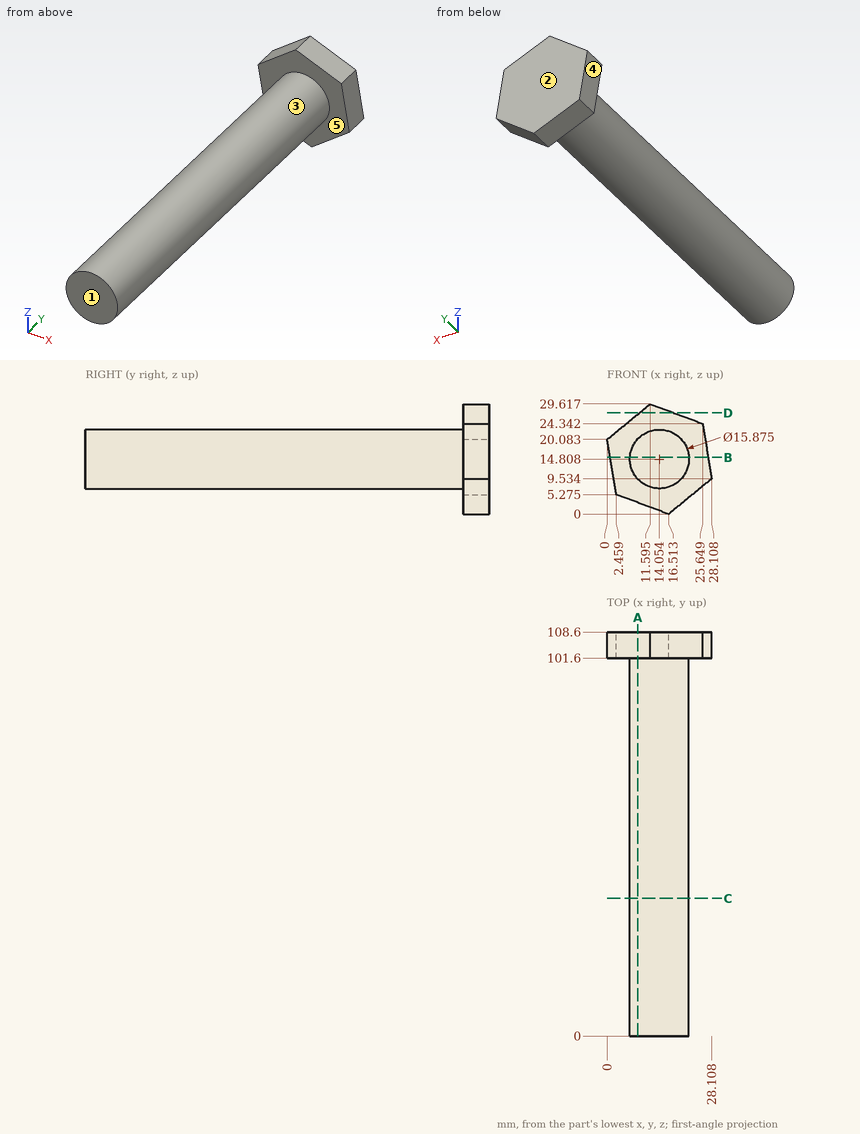
Drawing for the job (mm, zero at the part's lowest x, y, z). A direction names the side the tool comes from. Give positions to 0.01 mm unless a question says otherwise; leave off trailing zeros. Order: outer loops, then holes, each group sorted by start corner. A loop starts at its lowest first (then second) coordinate and runs counter-clockwise, first axis right, second up. Notation, with made-up numbers: M 71.5,4.25 L 76.5,4.25 A26 ccw 76.5,27.25 Z; hole C 66.5,74 d9. An arc over 180 degrees is marked long. Put each result on its own line as item: value.
Item 1: Probe line 1 (Y direction, x = 14.25, z = 28); line 2 (Z direction, x = 14, y = 13) (1 decimal); line 3 (Z direction, x = 18.5, y = 28) (1 decimal). List the from-to ranges inside material, lowest first. Write a range as [from, to].
From the geometry:
line 1: y = [101.6, 108.6]
line 2: z = [6.9, 22.7]
line 3: z = [8.2, 21.4]
Item 2: Slice it at C-C, the plane y = 37. Write the cut outline in (x, z) (1 decimal).
From the geometry:
outline: C 14.1,14.8 d15.9
Item 3: Two-plate mould, pull along Y, no slides. Class the marked faces 1, 2 and 3: +Y half, -Y half, draft (parallel to the pull), parting line (faces both ways), or undercut.
From the geometry:
face 1: -Y half
face 2: +Y half
face 3: draft
Item 4: 3-axis set-ups, long thin cutter, end or side, ignore diameter. For the marked faces 4 and 5: which of +Z, -Z, +X, -X, +Y, -Y reach the whole face in a straight line?
From the geometry:
face 4: -Z, -X, +Y, -Y
face 5: -Y
Item 5: Slice it at D-D, the plane z = 27.25. Write the cut outline in (x, y).
From the geometry:
outline: M 8.72,101.6 L 17.9,101.6 L 17.9,108.6 L 8.72,108.6 Z
Item 6: Flat gauge pins, fed straight in: pin 1 Ø6 at (x, y) = (7, 29) entering from -Z (1 decimal); pin 2 Ø6 at (y, z) = (15, 16.5) entering from -X; pin 3 Ø1 at (x, y) = (7.5, 47.5) entering from -Z (1 decimal); pin 4 Ø2 at (y, z) = (20.5, 25) entering from -X. Where does each tip first touch, or does it go through?
From the geometry:
pin 1: stops at z = 8
pin 2: stops at x = 6.12
pin 3: stops at z = 9.7
pin 4: passes through
Item 7: Slice it at B-B, the plane z = 15.25. Write the cut outline in (x, y), plus the area to 4 significant figures.
From the geometry:
outline: M 0.8,101.6 L 6.13,101.6 L 6.13,0 L 21.98,0 L 21.98,101.6 L 27.16,101.6 L 27.16,108.6 L 0.8,108.6 Z
area: 1,795 mm2
Item 8: Slice it at A-A, the plane x = 8.25. Write the cut outline in (y, z), plus the area to 3 significant figures.
From the geometry:
outline: M 0,9.39 L 101.6,9.39 L 101.6,3.1 L 108.6,3.1 L 108.6,26.87 L 101.6,26.87 L 101.6,20.22 L 0,20.22 Z
area: 1,270 mm2
